```python
from build123d import *

# Parameters (mm, degrees)
EXTRUDE_1_DEPTH     = 2
SKETCH_2_W          = 20
SKETCH_2_H          = 2
EXTRUDE_2_DEPTH     = 61.3
CUT_EXTRUDE_1_REACH = 79.504
SKETCH_4_R          = 3
CUT_EXTRUDE_2_REACH = 79.504
SKETCH_5_R          = 1.65


with BuildPart() as part:
    # 草图1 → 凸台-拉伸1 (new body)
    with BuildSketch(Plane.XY):
        with BuildLine():
            Line((0, 0), (0, 40))
            Line((0, 40), (20, 40))
            Line((20, 40), (20, 0))
            ThreePointArc((20, 0), (10, -10), (0, 0))
        make_face()
    extrude_1 = extrude(amount=EXTRUDE_1_DEPTH)

    # 草图2 → 凸台-拉伸2 (add)
    with BuildSketch(Plane.XY.offset(2)):
        with Locations((10, 39)):
            Rectangle(SKETCH_2_W, SKETCH_2_H)
    extrude(amount=EXTRUDE_2_DEPTH)

    # 镜向1: 凸台-拉伸1 across plane
    add(extrude_1.mirror(Plane.XY.offset(31.65)))

    # 草图4 → 切除-拉伸1 (cut, up to next)
    with BuildSketch(Plane.XY.offset(63.3), mode=Mode.PRIVATE) as cut_extrude_1_sk1:
        with Locations((10, 0)):
            Circle(SKETCH_4_R)
    cut_extrude_1_tool1 = extrude(cut_extrude_1_sk1.sketch, amount=-CUT_EXTRUDE_1_REACH, mode=Mode.PRIVATE) & part.part
    add(cut_extrude_1_tool1.solids().sort_by_distance((10, 0, 63.3))[0], mode=Mode.SUBTRACT)

    # 草图5 → 切除-拉伸2 (cut, up to next)
    with BuildSketch(Plane(origin=(0, 0, 0), x_dir=(-1, 0, 0), z_dir=(0, 0, -1)), mode=Mode.PRIVATE) as cut_extrude_2_sk1:
        with Locations((-10, -7)):
            Circle(SKETCH_5_R)
    cut_extrude_2_tool1 = extrude(cut_extrude_2_sk1.sketch, amount=-CUT_EXTRUDE_2_REACH, mode=Mode.PRIVATE) & part.part
    # 草图5 → 切除-拉伸2 (cut, up to next)
    with BuildSketch(Plane(origin=(0, 0, 0), x_dir=(-1, 0, 0), z_dir=(0, 0, -1)), mode=Mode.PRIVATE) as cut_extrude_2_sk2:
        with Locations((-17, 0)):
            Circle(SKETCH_5_R)
    cut_extrude_2_tool2 = extrude(cut_extrude_2_sk2.sketch, amount=-CUT_EXTRUDE_2_REACH, mode=Mode.PRIVATE) & part.part
    # 草图5 → 切除-拉伸2 (cut, up to next)
    with BuildSketch(Plane(origin=(0, 0, 0), x_dir=(-1, 0, 0), z_dir=(0, 0, -1)), mode=Mode.PRIVATE) as cut_extrude_2_sk3:
        with Locations((-10, 7)):
            Circle(SKETCH_5_R)
    cut_extrude_2_tool3 = extrude(cut_extrude_2_sk3.sketch, amount=-CUT_EXTRUDE_2_REACH, mode=Mode.PRIVATE) & part.part
    # 草图5 → 切除-拉伸2 (cut, up to next)
    with BuildSketch(Plane(origin=(0, 0, 0), x_dir=(-1, 0, 0), z_dir=(0, 0, -1)), mode=Mode.PRIVATE) as cut_extrude_2_sk4:
        with Locations((-3, 0)):
            Circle(SKETCH_5_R)
    cut_extrude_2_tool4 = extrude(cut_extrude_2_sk4.sketch, amount=-CUT_EXTRUDE_2_REACH, mode=Mode.PRIVATE) & part.part
    add(cut_extrude_2_tool1.solids().sort_by_distance((10, -7, 0))[0], mode=Mode.SUBTRACT)
    add(cut_extrude_2_tool2.solids().sort_by_distance((17, 0, 0))[0], mode=Mode.SUBTRACT)
    add(cut_extrude_2_tool3.solids().sort_by_distance((10, 7, 0))[0], mode=Mode.SUBTRACT)
    add(cut_extrude_2_tool4.solids().sort_by_distance((3, 0, 0))[0], mode=Mode.SUBTRACT)


solid = part.part
```
CAD build for the part. Positions are in the model's coordinates, mm. A direction names the side the tool comes from. Round coordinates to 2 decimals unless told otherwise and drop trailing zeros. Write each loop counter-clockwise with the first axis right and the second up, starting at its lowest first coordinate (ties: lowest second). Pieces come first, ordered by that corner, then holes. Notation, with made-up numbers: (77.25, 66) -> (106.25, 66) arc R27 ccw to (106.25, 90) -> close; hole circle Ø10 at (22, 76). An arc over 180 degrees is marked (long way). Answer in a Markdown table with one row per item. Add a question column.
Item 1: Saw through at C-C, the plane y = 7. Write the cut outline in (x, z).
Item 2: Mould opens along X. For faces 5 (the face through (8.476, -7.632, 0.986)), 6 (the face through (0, 39, 32)), 7 (the face through (10, 14, 2)) say: pulls with the +X half, pulls with the -X half, needs draft (parallel to the pull), parting line crosses it, or undercut.
Item 3: Saw through at A-A, the plane y = 13. Write the cut outline in (x, z).
Item 4: Saw through at D-D, the plane x = 2.25. Write the cut outline in (y, z).
Item 5: Drill centre lines: line 1 (Y direction, x = 10, z = 0.6); line 2 (Z direction, x = 3.75, y = 3.5); line 3 (Y direction, x = 18, z = 17.5). Where is each one in solid material? Low to high. Write a range as from..to.
Item 6: Which spindle directions (+Z, -Z, +X, -X, +Y, -Y) get a long thin tool onto all of the face, cutting with end or side? Do faces 1 (the face through (15.476, -0.632, 0.986)), 2 (the face through (10, 38, 31)), 3 (the face through (12.77, -1.15, 62.31)), 4 (the face through (10, 15, 0)). Say none if no direction does.
Item 7: Drop flat-ended pins along their axis: pin 1 Ø1 at (x, z) = (14.5, 39) entering from -Y; pin 2 Ø2 at (x, y) = (10, 7) entering from -Z. Give the stop position or say it passes through.
Item 8: Saw through at B-B, the plane x = 10. Write the cut outline in (y, z).
Findings below:
| question | item | result |
|---|---|---|
| 1 | outline | (0, 0) -> (8.35, 0) -> (8.35, 2) -> (0, 2) -> close; (0, 61.3) -> (20, 61.3) -> (20, 63.3) -> (0, 63.3) -> close; (11.65, 0) -> (20, 0) -> (20, 2) -> (11.65, 2) -> close |
| 2 | face 5 | undercut |
| 2 | face 6 | pulls with the -X half |
| 2 | face 7 | needs draft |
| 3 | outline | (0, 0) -> (20, 0) -> (20, 2) -> (0, 2) -> close; (0, 61.3) -> (20, 61.3) -> (20, 63.3) -> (0, 63.3) -> close |
| 4 | outline | (-6.32, 0) -> (-1.47, 0) -> (-1.47, 2) -> (-6.32, 2) -> close; (-6.32, 61.3) -> (38, 61.3) -> (38, 2) -> (1.47, 2) -> (1.47, 0) -> (40, 0) -> (40, 63.3) -> (-6.32, 63.3) -> close |
| 5 | line 1 | y = -10..-8.65, -5.35..5.35, 8.65..40 |
| 5 | line 2 | z = 0..2, 61.3..63.3 |
| 5 | line 3 | y = 38..40 |
| 6 | face 1 | -Z |
| 6 | face 2 | +X, -X, -Y |
| 6 | face 3 | +Z |
| 6 | face 4 | -Z, +X, -X, +Y, -Y |
| 7 | pin 1 | stops at y = 38 |
| 7 | pin 2 | stops at z = 61.3 |
| 8 | outline | (-10, 0) -> (-8.65, 0) -> (-8.65, 2) -> (-10, 2) -> close; (-10, 61.3) -> (-3, 61.3) -> (-3, 63.3) -> (-10, 63.3) -> close; (-5.35, 0) -> (5.35, 0) -> (5.35, 2) -> (-5.35, 2) -> close; (3, 61.3) -> (38, 61.3) -> (38, 2) -> (8.65, 2) -> (8.65, 0) -> (40, 0) -> (40, 63.3) -> (3, 63.3) -> close |
